Read the model definition and answer for the solid it produces. Units are mm, in the model's axes. A direction names the side the tool comes from. Round coordinates to 2 decimals unless told otherwise and drop trailing zeros. Order: outer loops, then holes, each group sorted by start corner. A loop starts at its lowest first (then second) coordinate and runs counter-clockwise, first axis right, second up. Notation, with made-up numbers: (64.25, -1.5) - (69.25, -1.5) arc R16 cw to (69.25, 26.5) - close; hole circle Ø2 at (-11, 50.25). An arc over 180 degrees is marked (long way). One line per question, with ' | ' between items. Start each with the question number.
1) The part is cut by section C-C, the plane x = 0.65. Count the separate pieces of the cut face and the enclosed holes in it, plus the area to 3 significant figures.
2) The mould has two halves that part along Z. Classify faces 4 (the cylindrical face through (1.252, -8.103, -21.909)), 5 (the flat face through (1.25, -19.45, -116.6)), 6 (the flat face through (0, -10, -73)): pulls with the +Z half, pulls with the -Z half, needs draft (parallel to the pull), parting line crosses it, or undercut.
3) The part is cut by section B-B, the plane z = -77. Give the vertices of the cut face in (x, y), plus the area to 3 significant figures.
4) Flat-ended cylindrical pins translate along their axes: pin 1 (0.6 mm diameter, centred on x = 1.5, y = 7, fed in from -Z); pin 2 (12 mm diameter, centred on y = -23, z = -32, fed in from +X); pin 3 (0.8 mm diameter, centred on x = 1.5, z = -14, fed in from +Y); pin 4 (0.8 mm diameter, centred on x = 1, z = -32, fed in from -Y). Find the tip coordinate at first contact, or state that the pin passes through.
5) Straight lines are drawn through the part: line 1 (Z direction, x = 2.2, y = 0.5); line 2 (Z direction, x = 2.4, y = -7.5); line 3 (Y direction, x = 0.4, z = -96). For each, find the intervals that lie inside material, in ascending order. Write a range as from..to.
6) For faces 1 (the cylindrical face through (1.25, -2.72, -118.83)), 2 (the cylindrical face through (1.25, 11.55, -6.43)), 3 (the cylindrical face through (1.29, 13.77, -98.73)), determine the directions among +Z, -Z, +X, -X, +Y, -Y from which every point of the face is accessible in a straight line to the end or side of a thin tool.
7) The part is cut by section A-A, the plane z = -12. Give the vertices of the cut face in (x, y).
8) The part is cut by section D-D, the plane z = -45.5. Give the vertices of the cut face in (x, y).
Autodesk Inventor part; units mm, degrees
ref_plane "Work Plane2" through (0, -42.6838, -105.8119) normal (0, -0.8661, 0.4999) x (1, 0, 0)
ref_plane "YZ Plane" through (0, 0, 0) normal (1, 0, 0) x (0, 1, 0)
ref_plane "XZ Plane" through (0, 0, 0) normal (0, 1, 0) x (-1, 0, 0)
sketch "Sketch1" plane through (0, 0, 0) normal (1, 0, 0) x (0, 1, 0)
  line L0 (14.231, -0.0045) -> (14.2475, -121.0044)
  circle A0 centre (46.8483, -60.5) radius 44
  arc A1 (-10.6283, -58.8604) -> (-0.114, -93.6782) centre (46.8483, -60.5) ccw
  line L1 (-0.114, -93.6782) -> (2.9975, -94.9709)
  arc A2 (2.9975, -94.9709) -> (7.0992, -99.6298) centre (46.8483, -60.5) ccw
  line L2 (7.0992, -99.6298) -> (13.2859, -93.5395)
  arc A3 (-0.2275, -59.1156) -> (13.2859, -93.5395) centre (46.8483, -60.5) ccw
  line L3 (-0.2275, -59.1156) -> (-8.9052, -58.8604)
  line L4 (-8.9052, -58.8604) -> (-10.6283, -58.8604)
  circle A4 centre (84.1308, -7.2551) radius 2.15
  circle A5 centre (95.3483, -109) radius 2.65
  circle A6 centre (100.0932, -97.7825) radius 2.15
  circle A7 centre (-6.3966, -23.2175) radius 2.15
  circle A8 centre (-6.3966, -97.7825) radius 2.15
  circle A9 centre (-1.6517, -12) radius 2.65
  circle A10 centre (95.3483, -12) radius 2.65
  circle A11 centre (9.5658, -113.7449) radius 2.15
  circle A12 centre (9.5658, -7.2551) radius 2.15
  circle A13 centre (84.1308, -113.7449) radius 2.15
  circle A14 centre (100.0932, -23.2175) radius 2.15
  circle A15 centre (-1.6517, -109) radius 2.65
  line L5 (-7.7476, -49.0794) -> (0.7499, -50.8569)
  arc A16 (12.1591, -28.6456) -> (0.7499, -50.8569) centre (46.8483, -60.5) ccw
  line L6 (12.1591, -28.6456) -> (5.7646, -22.7737)
  arc A17 (5.7646, -22.7737) -> (-7.7476, -49.0794) centre (46.8483, -60.5) ccw
  line L7 (83.7453, -102.33) -> (78.0025, -95.8194)
  arc A18 (66.2911, -103.3955) -> (78.0025, -95.8194) centre (46.8483, -60.5) ccw
  line L8 (66.2911, -103.3955) -> (69.8751, -111.3026)
  arc A19 (69.8751, -111.3026) -> (83.7453, -102.33) centre (46.8483, -60.5) ccw
  line L9 (85.3896, -20.1799) -> (79.3909, -26.4555)
  arc A20 (89.1056, -39.7066) -> (79.3909, -26.4555) centre (46.8483, -60.5) ccw
  line L10 (89.1056, -39.7066) -> (96.8951, -35.8737)
  arc A21 (96.8951, -35.8737) -> (85.3896, -20.1799) centre (46.8483, -60.5) ccw
  line L11 (58.0786, -115.1353) -> (56.3307, -106.6317)
  arc A22 (42.4628, -107.3915) -> (56.3307, -106.6317) centre (46.8483, -60.5) ccw
  line L12 (42.4628, -107.3915) -> (41.6544, -116.0352)
  arc A23 (41.6544, -116.0352) -> (58.0786, -115.1353) centre (46.8483, -60.5) ccw
  line L13 (11.1274, -17.6613) -> (16.6872, -24.3288)
  arc A24 (31.0571, -16.1301) -> (16.6872, -24.3288) centre (46.8483, -60.5) ccw
  line L14 (31.0571, -16.1301) -> (28.1463, -7.9512)
  arc A25 (28.1463, -7.9512) -> (11.1274, -17.6613) centre (46.8483, -60.5) ccw
  line L15 (101.6271, -71.0083) -> (93.1011, -69.3728)
  arc A26 (82.2782, -91.5285) -> (93.1011, -69.3728) centre (46.8483, -60.5) ccw
  line L16 (82.2782, -91.5285) -> (88.8092, -97.2481)
  arc A27 (88.8092, -97.2481) -> (101.6271, -71.0083) centre (46.8483, -60.5) ccw
  line L17 (100.5451, -45.4072) -> (92.1875, -47.7563)
  arc A28 (93.8596, -63.3257) -> (92.1875, -47.7563) centre (46.8483, -60.5) ccw
  line L18 (93.8596, -63.3257) -> (102.5254, -63.8466)
  arc A29 (102.5254, -63.8466) -> (100.5451, -45.4072) centre (46.8483, -60.5) ccw
  line L19 (38.2646, -115.6131) -> (39.6006, -107.0351)
  arc A30 (20.5997, -99.6032) -> (39.6006, -107.0351) centre (46.8483, -60.5) ccw
  line L20 (20.5997, -99.6032) -> (15.7612, -106.8113)
  arc A31 (15.7612, -106.8113) -> (38.2646, -115.6131) centre (46.8483, -60.5) ccw
  line L21 (38.8508, -5.2987) -> (40.0955, -13.8905)
  arc A32 (56.4914, -14.4016) -> (40.0955, -13.8905) centre (46.8483, -60.5) ccw
  line L22 (56.4914, -14.4016) -> (58.2689, -5.9041)
  arc A33 (58.2689, -5.9041) -> (38.8508, -5.2987) centre (46.8483, -60.5) ccw
  arc A34 (6.34, -0.0055) -> (-13.6572, -20.0083) centre (6.3428, -20.0055) ccw
  line L23 (6.34, -0.0055) -> (87.34, 0.0055)
  arc A35 (107.3428, -19.9917) -> (87.34, 0.0055) centre (87.3428, -19.9945) ccw
  line L24 (107.3428, -19.9917) -> (107.3538, -100.9917)
  arc A36 (87.3566, -120.9945) -> (107.3538, -100.9917) centre (87.3538, -100.9945) ccw
  line L25 (87.3566, -120.9945) -> (6.3566, -121.0055)
  arc A37 (-13.6462, -101.0083) -> (6.3566, -121.0055) centre (6.3538, -101.0055) ccw
  line L26 (-13.6462, -101.0083) -> (-13.6572, -20.0083)
  line L27 (-13.651, -65.8198) -> (-34.151, -83.0261)
  line L28 (-34.151, -83.0261) -> (-46.1481, -103.8124)
  line L29 (-46.1481, -103.8124) -> (-46.1481, -112.3124)
  line L30 (-46.1481, -112.3124) -> (-36.5178, -121.0114)
  line L31 (-36.5178, -121.0114) -> (-13.6462, -101.0083)
  circle A38 centre (46.8483, -60.5) radius 50
  circle A39 centre (-1.6517, -109) radius 5.75
  line L32 (-69.3325, -76.5758) -> (-2.1613, -115.3449)
  line L33 (-36.5178, -121.0114) -> (-29.7828, -121.0105)
  line L34 (-29.7828, -121.0105) -> (-1.6517, -109)
  point P0 (0, 0)
  point P1 (14.2445, -98.4076)
  point P2 (14.2341, -22.6013)
  point P3 (-9.9753, -112.5537)
  dimension "d4" = 100
  dimension "d5" = 60
  dimension "d6" = 90
  dimension "d7" = 12
  dimension "d8" = 12
  dimension "d26" = 8.5
  dimension "d27" = 20.5
  dimension "d29" = 0
  dimension "d36" = 50
extrude "Extrusion1" add sketch "Sketch1" along normal blind 2.54 contours L34 A39 L32 | L0 A25 L13 A38 L6 A17 L5 L3 L4 A1 L1 A2 L2 L25 A37 L34 L32 L26 A34 L23 | L0 L13 A25 | L26 L31 L32 L28 L27 | A38 L5 A17 L6 | A37 L32 L31 | L32 L34 A37 | A37 L34 L33 L31 L32 | L31 L30 L29 L28 L32 | A38 L2 A2 L1 A1 L4 L3 | A39
fillet "Fillet1" radius 6 4 edges at (1.27, 14.231, -0.0045) (1.27, 14.2475, -121.0044) (1.27, 14.2445, -98.4076) (1.27, 14.2341, -22.6013)
sketch "Sketch3" plane through (0, 0, 0) normal (-1, 0, 0) x (0, 0, 1)
  circle A0 centre (-12, -1.6517) radius 2.65
  circle A1 centre (-12, -1.6517) radius 4.05
  circle A2 centre (-109, -1.6517) radius 2.65
  circle A3 centre (-109, -1.6517) radius 4.05
  point P0 (0, 0)
  dimension "d13" = 8.1
  dimension "d14" = 8.1
extrude "Extrusion3" cut sketch "Sketch3" against normal through all contours A0 | A1 | A2 | A3
ref_plane "Work Plane2" through (0, -42.6838, -105.8119) normal (0, -0.8661, 0.4999) x (1, 0, 0)
sketch "Sketch4" plane through (0, -42.6838, -105.8119) normal (0, -0.8661, 0.4999) x (1, 0, 0)
  circle A0 centre (-17.46, 13) radius 21
  line L0 (0, 24) -> (0, 0)
  line L1 (0, 24) -> (2.54, 24)
  line L2 (0, 49.1499) -> (0, 24)
  line L3 (0, 0) -> (0, -7.3618)
  line L4 (0, 1.3317) -> (3.4521, 1.3317)
  line L5 (3.4521, 1.3317) -> (7.9852, 19.2714)
  line L6 (0, 24.6683) -> (6.7025, 24.6683)
  line L7 (6.7025, 24.6683) -> (7.9852, 19.2714)
  line L8 (0, 13.7) -> (2.54, 13.7)
  line L9 (0, 11.3553) -> (2.54, 11.3553)
  line L10 (0, 11.3553) -> (0, 30.1698)
  point P0 (0, 112.9799)
  point P1 (0.4285, 24)
  point P2 (0, 24.6683)
  dimension "d18" = 42
  dimension "d19" = 17.46
  dimension "d30" = 0.7
extrude "Extrusion4" cut sketch "Sketch4" against normal blind 7.1 contours L6 L7 L5 L4 A0 | A0 L1 L2 | L0 L1 A0
sketch "Sketch5" plane through (0, 0, 0) normal (-1, 0, 0) x (0, 0, 1)
  circle A0 centre (-114.2363, -33.5753) radius 2.65
  line L0 (-112.3124, -46.1481) -> (-121.0114, -36.5178)
  line L1 (-108.2077, -35.8688) -> (-87.996, -24.2033)
  point P0 (0, 0)
  point P1 (-88.5749, -24.5372)
  dimension "d23" = 5.3
  dimension "d24" = 7
  dimension "d25" = 5
extrude "Extrusion5" cut sketch "Sketch5" against normal through all
sketch "Sketch6" plane through (0, 0, 0) normal (-1, 0, 0) x (0, 0, 1)
  circle A0 centre (-77, -19.6494) radius 1.6
  line L0 (-20.0083, -13.6572) -> (-65.8198, -13.651)
  circle A1 centre (-109, -1.6517) radius 4.05
  point P0 (0, 0)
  dimension "d33" = 3.2
  dimension "d34" = 6
  dimension "d35" = 32
extrude "Extrusion6" cut sketch "Sketch6" against normal through all contours A0
fillet "Fillet2" radius 6 5 edges at (1.27, -34.151, -83.0261) (1.27, -46.1481, -103.8124) (1.27, -46.1481, -112.3124) (1.27, -36.5178, -121.0114) (1.27, -29.7828, -121.0105)
properties part number "output_support"
Values:
1) separate pieces: 1 | enclosed holes: 9 | area: 3,120 mm^2
2) face 4: undercut | face 5: pulls with the -Z half | face 6: needs draft
3) outline: (0, -26.97) - (2.54, -26.97) - (2.54, -21.25) - (0, -21.25) - close; (0, -18.05) - (2.54, -18.05) - (2.54, -0.35) - (0, -0.35) - close | area: 59.5 mm^2
4) pin 1: stops at z = -121.01 | pin 2: passes through | pin 3: stops at y = 14.23 | pin 4: stops at y = -13.66
5) line 1: z = -120.13..-112.43, -105.57..-79.26, -41.74..-15.43, -8.57..-0.88 | line 2: z = -115.43..-99.63, -95.94..-25.06, -21.37..-5.57 | line 3: y = -41.64..-37.02, -28.82..-7.6, -5.19..11.64
6) face 1: -Z, +X, -X | face 2: +X, -X | face 3: +X, -X, +Y
7) outline: (0, -11.99) - (2.54, -11.99) - (2.54, -5.7) - (0, -5.7) - close; (0, 2.4) - (2.54, 2.4) - (2.54, 14.23) - (0, 14.23) - close
8) outline: (0, -13.65) - (2.54, -13.65) - (2.54, -0.85) - (0, -0.85) - close
